Here's the drawing with two shaded views (mm, measured from the low corner). I have some questions. A direction names the side the tool comes from. Round coordinates to 2 decimals unless told otherwise and drop trailing zeros. Order: outer loops, then holes, each group sorted by start corner. A loop starts at its lowest first (then second) coordinate and runs counter-clockwise, first axis right, second up.
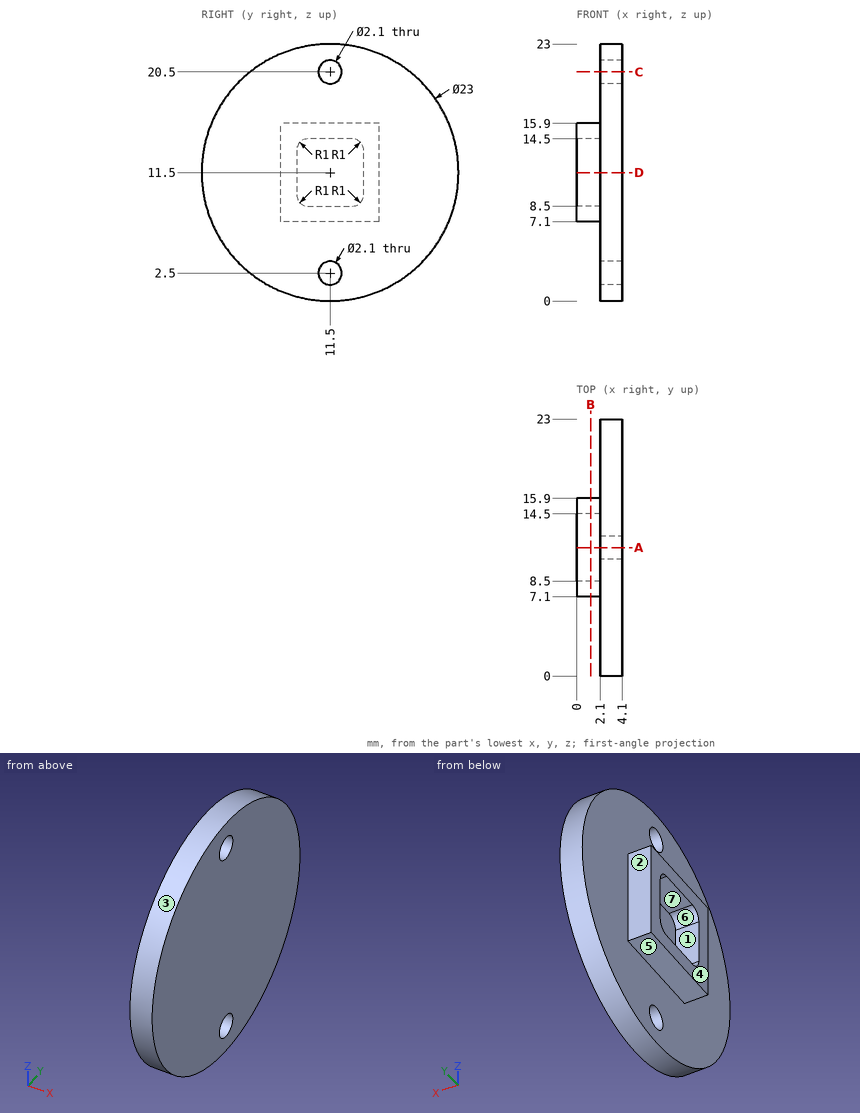
1. I need wall thicknesses on probe 1 along Z at (x, y) = (3.3, 11.5); probe 2 along Y at (x, z) = (0.35, 9.75); probe 3 along X at (y, z) = (17, 15.25). Which ranges of each line are inside material? Lowest first, please.
Evaluation:
probe 1: z = 0 to 1.45, 3.55 to 19.45, 21.55 to 23
probe 2: y = 7.1 to 8.5, 14.5 to 15.9
probe 3: x = 2.1 to 4.1
2. If we section it at D-D, the plane z = 11.5: Write out the boundary of the cut face in (x, y), and give its area (3 significant figures).
Evaluation:
outline: (0, 7.1) - (2.1, 7.1) - (2.1, 0) - (4.1, 0) - (4.1, 23) - (2.1, 23) - (2.1, 15.9) - (0, 15.9) - (0, 14.5) - (2.1, 14.5) - (2.1, 8.5) - (0, 8.5) - close
area: 51.9 mm2
3. If we section it at C-C, the plane z = 20.5: Write out the boundary of the cut face in (x, y), and give its area (3 significant figures).
Evaluation:
outline: (2.1, 4.34) - (4.1, 4.34) - (4.1, 10.45) - (2.1, 10.45) - close; (2.1, 12.55) - (4.1, 12.55) - (4.1, 18.66) - (2.1, 18.66) - close
area: 24.4 mm2
4. On a 3-axis mill with a long thin cutter (end or side, diameter ignored), from which of +Z, -Z, +X, -X, +Y, -Y can I reach the whole of each face in a straight line? I mean the marked faces 1, 2 and 3. Say none if no direction works.
Evaluation:
face 1: -X
face 2: +Z, -Z, -X, +Y
face 3: +X, -X
5. I'm going to push flat-ended pins straight in: P1, Ø1.7, axis at x = 1.5, z = 10, coming from the +Y side; P2, Ø0.6, axis at x = 1, y = 12, coming from the -Z side; P3, Ø6.5, axis at y = 11, z = 12, coming from the -X side; P4, Ø1.5, axis at x = 2, z = 5, coming from the -Y side. Where does each tip first touch, or does it pass through?
Evaluation:
P1: stops at y = 22.96
P2: stops at z = 7.1
P3: stops at x = 0
P4: stops at y = 1.54
6. If we section it at A-A, the plane y = 11.5: Write out the boundary of the cut face in (x, z).
Evaluation:
outline: (0, 7.1) - (2.1, 7.1) - (2.1, 3.55) - (4.1, 3.55) - (4.1, 19.45) - (2.1, 19.45) - (2.1, 15.9) - (0, 15.9) - (0, 14.5) - (2.1, 14.5) - (2.1, 8.5) - (0, 8.5) - close; (2.1, 0) - (4.1, 0) - (4.1, 1.45) - (2.1, 1.45) - close; (2.1, 21.55) - (4.1, 21.55) - (4.1, 23) - (2.1, 23) - close
7. If we mould it in two halves opening along Z, with no side actions, what happens to the marked faces 4, 5, 6 and 7? For each: released by +Z, released by -Z, zero draft, split by the parting line, or undercut.
Evaluation:
face 4: zero draft
face 5: released by -Z
face 6: undercut
face 7: undercut
8. If we section it at B-B, the plane x = 1.25: Write out the boundary of the cut face in (y, z), and give its area (3 significant figures).
Evaluation:
outline: (7.1, 7.1) - (15.9, 7.1) - (15.9, 15.9) - (7.1, 15.9) - close; hole (8.5, 9.5) arc R1 ccw to (9.5, 8.5) - (13.5, 8.5) arc R1 ccw to (14.5, 9.5) - (14.5, 13.5) arc R1 ccw to (13.5, 14.5) - (9.5, 14.5) arc R1 ccw to (8.5, 13.5) - close
area: 42.3 mm2
